The model under review builds one solid part; all positions refer to its coordinate system, in mm. Coordinates: 2 decimals unless noted, no trailing zeros. Write each loop counter-clockwise with the first axis right and the second up, starting at its lowest first coordinate (ties: lowest second). Pieces come first, ordered by that corner, then holes. Notation, with made-up numbers: (-1, 34.25) - (18, 34.25) arc R31 ccw to (18, 61.25) - close; hole circle Ø5 at (54, -2.5). An arc over 180 degrees is marked (long way). Use one line per item in the form item = value. Start each with the question number.
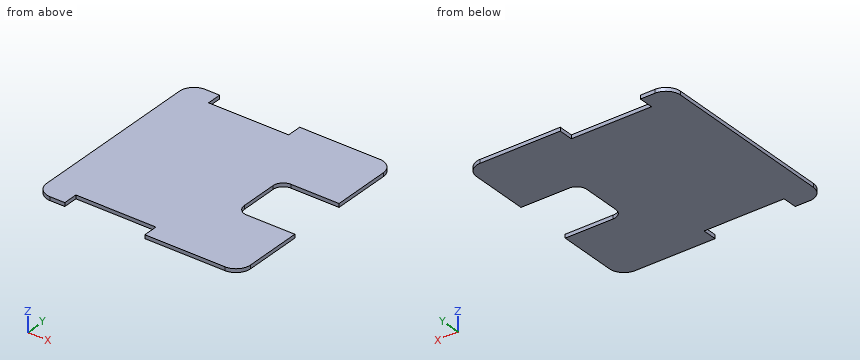
```python
from build123d import *

# Parameters (mm, degrees)
BOSS_EXTRUDE1_DEPTH = 6.35
SKETCH2_W           = 139.7
SKETCH2_H           = 25.4
CUT_EXTRUDE1_DEPTH  = 503.934431611
CUT_EXTRUDE2_DEPTH  = 503.934431611


with BuildPart() as part:
    # Sketch1 → Boss-Extrude1 (new body)
    with BuildSketch(Plane.XY):
        with BuildLine():
            Line((25.4, 0), (330.2, 0))
            ThreePointArc((330.2, 0), (348.160512242, 7.439487758), (355.6, 25.4))
            Line((355.6, 25.4), (355.6, 330.2))
            ThreePointArc((355.6, 330.2), (348.160512242, 348.160512242), (330.2, 355.6))
            Line((330.2, 355.6), (25.4, 355.6))
            ThreePointArc((25.4, 355.6), (7.439487758, 348.160512242), (0, 330.2))
            Line((0, 330.2), (0, 25.4))
            ThreePointArc((0, 25.4), (7.439487758, 7.439487758), (25.4, 0))
        make_face()
    extrude(amount=BOSS_EXTRUDE1_DEPTH)

    # Sketch2 → Cut-Extrude1 (cut, through all)
    with BuildSketch(Plane(origin=(0, 0, 0), x_dir=(-1, 0, 0), z_dir=(0, 0, -1))):
        with Locations((-120.65, 342.9)):
            Rectangle(SKETCH2_W, SKETCH2_H)
        with Locations((-120.65, 12.7)):
            Rectangle(SKETCH2_W, SKETCH2_H)
    extrude(amount=-CUT_EXTRUDE1_DEPTH, mode=Mode.SUBTRACT)

    # Sketch3 → Cut-Extrude2 (cut, through all)
    with BuildSketch(Plane(origin=(0, 0, 0), x_dir=(-1, 0, 0), z_dir=(0, 0, -1))):
        with BuildLine():
            Line((-355.6, 127), (-271.78, 127))
            ThreePointArc((-271.78, 127), (-259.207641431, 132.207641431), (-254, 144.78))
            Line((-254, 144.78), (-254, 210.82))
            ThreePointArc((-254, 210.82), (-259.207641431, 223.392358569), (-271.78, 228.6))
            Line((-271.78, 228.6), (-355.6, 228.6))
            Line((-355.6, 228.6), (-355.6, 127))
        make_face()
    extrude(amount=-CUT_EXTRUDE2_DEPTH, mode=Mode.SUBTRACT)


solid = part.part
```
1. Take a section at A-A (x = 321.5). State the section outline as (y, z) points.
2. Take a section at D-D (x = 114). State the section outline as (y, z) points, plus the area to 3 significant figures.
3. Take a section at C-C (y = 168). State the section outline as (x, z) points.
4. For P1, Ø1.9, axis at y = 18, z = 3, coming from the -X side; P2, Ø3, axis at y = 162.5, z = 3.5, coming from the +X side; P3, Ø3, axis at y = 344.5, z = 4.5, coming from the +X side, all flat-tipped, find the tip position at first contact; note any pin that passes through.
5. For L1, parallel to X at y = 24.5, z = 3.25; L2, parallel to Y at x = 317.5, z = 2.5; L3, parallel to Y at x = 256, z = 0.75, list the stretches that pass through material, from the lowest coordinate up.
6. Take a section at B-B (z = 4.75). State the section outline as (x, y) points.
Returned:
q1.outline = (0, 0) - (127, 0) - (127, 6.35) - (0, 6.35) - close; (228.6, 0) - (355.6, 0) - (355.6, 6.35) - (228.6, 6.35) - close
q2.outline = (25.4, 0) - (330.2, 0) - (330.2, 6.35) - (25.4, 6.35) - close
q2.area = 1,940 mm²
q3.outline = (0, 0) - (254, 0) - (254, 6.35) - (0, 6.35) - close
q4.P1 = 0.83
q4.P2 = 254
q4.P3 = 352.14
q5.L1 = 0.02 to 50.8, 190.5 to 355.58
q5.L2 = 0 to 127, 228.6 to 355.6
q5.L3 = 0 to 136.59, 219.01 to 355.6
q6.outline = (0, 25.4) arc R25.4 ccw to (25.4, 0) - (50.8, 0) - (50.8, 25.4) - (190.5, 25.4) - (190.5, 0) - (330.2, 0) arc R25.4 ccw to (355.6, 25.4) - (355.6, 127) - (271.78, 127) arc R17.78 cw to (254, 144.78) - (254, 210.82) arc R17.78 cw to (271.78, 228.6) - (355.6, 228.6) - (355.6, 330.2) arc R25.4 ccw to (330.2, 355.6) - (190.5, 355.6) - (190.5, 330.2) - (50.8, 330.2) - (50.8, 355.6) - (25.4, 355.6) arc R25.4 ccw to (0, 330.2) - close
